Work out the finished part from the listing and answer in its coordinate system (mm). Coordinates: 2 decimals unless noted, no trailing zeros. Write each loop counter-clockwise with the first axis right and the second up, starting at its lowest first coordinate (ties: lowest second). Pieces come first, ordered by that corner, then holes. Notation, with made-up numbers: (-38.75, -16) - (-18.75, -16) arc R15 cw to (-18.75, -5) - close; hole circle Ø5 at (44, 85). An arc over 180 degrees is marked (long way). One line per item, written item: value.
```python
from build123d import *

# Parameters (mm, degrees)
SKETCH1_W = 70
SKETCH1_H = 3


with BuildPart() as part:
    # Sketch1 → Revolve1 (revolve)
    with BuildSketch(Plane.XY, mode=Mode.PRIVATE) as revolve1_sk:
        Rectangle(SKETCH1_W, SKETCH1_H)
    revolve(revolve1_sk.sketch.rotate(Axis((-35, 1.5, 0), (1, 0, 0)), 270), axis=Axis((-35, 1.5, 0), (1, 0, 0)))

    # Sketch2 → Revolve2 (revolve)
    with BuildSketch(Plane.XY, mode=Mode.PRIVATE) as revolve2_sk:
        Polygon((-44, 1.445289322), (-37, 1.445736138), (-37, 10.445863799), (-44, 10.445863799), align=None)
        with BuildLine():
            Line((-37, 10.445863799), (-37, 1.445736138))
            Line((-37, 1.445736138), (-35, 1.445863799))
            Line((-35, 1.445863799), (-35, 8.445863799))
            ThreePointArc((-35, 8.445863799), (-35.585786438, 9.860077362), (-37, 10.445863799))
        make_face()
        with BuildLine():
            Line((-50, 1.444906337), (-44, 1.445289322))
            Line((-44, 1.445289322), (-44, 10.445863799))
            ThreePointArc((-44, 10.445863799), (-48.242640687, 8.688504486), (-50, 4.445863799))
            Line((-50, 4.445863799), (-50, 1.444906337))
        make_face()
    revolve2 = revolve(revolve2_sk.sketch.rotate(Axis((-50, 1.444906337, 0), (0.9999999979628139, 6.383080945348042e-05, 0)), 180), axis=Axis((-50, 1.444906337, 0), (0.9999999979628139, 6.383080945348042e-05, 0)))

    # Mirror1: Revolve2 across plane
    add(revolve2.mirror(Plane(origin=(0, 0, 0), x_dir=(0, 0, 1), z_dir=(1, 0, 0))))


solid = part.part
```
Item 1: Given pin 1 (1.5 mm diameter, centred on x = -39, y = -3.5, fed in from -Z); pin 2 (8 mm diameter, centred on x = -16.5, z = 2.5, fed in from -Y); pin 3 (6 mm diameter, centred on x = 16, y = 2.5, fed in from +Z), each flat-ended and moving along its own axis, determine where each tip first touches the part or whether it passes through.
Evaluation:
pin 1: stops at z = -7.96
pin 2: stops at y = -1.5
pin 3: stops at z = 3
Item 2: Determine the mould class of faces 1 (the face through (50, 1, 0)), 2 (the face through (-50, 1, 0)), 3 (the face through (35, 2.1, 3.1)) for opening direction X: +X half, -X half, draft (parallel to the pull), parting line (faces both ways), or undercut.
Evaluation:
face 1: +X half
face 2: -X half
face 3: undercut
Item 3: Consider probe 1 along Z at (x, y) = (24, 1.75); probe 2 along X at (y, z) = (-3.25, 6); probe 3 along X at (y, z) = (5.25, 2.5). Determine where each line is inside the solid, lowest interval first.
Evaluation:
probe 1: z = -2.99 to 2.99
probe 2: x = -47.83 to -35.1, 35.1 to 47.83
probe 3: x = -49.8 to -35, 35 to 49.8
Item 4: Section A-A, the plane x = -7 is taken. Determine the outline of the cut face in (y, z).
Evaluation:
outline: circle Ø6 at (1.5, 0)
